```python
from build123d import *

# Parameters (mm, degrees)
F0_W     = 76.2
F0_H     = 50.8
F1_DEPTH = 2.54
F2_W     = 71.12
F2_H     = 45.72
F3_DEPTH = 2.54
F4_W     = 33.02
F4_H     = 5.08
F5_DEPTH = 2.54
F7_DEPTH = 2.54
F9_DEPTH = 25.4


with BuildPart() as f1:
    # F0 (on Top) → F1 (new body)
    with BuildSketch(Plane.XY):
        with Locations((13.626695, -1.068337)):
            Rectangle(F0_W, F0_H)
    extrude(amount=F1_DEPTH)

    # F2 (on face) → F3 (join)
    with BuildSketch(Plane.XY.offset(2.54)):
        with Locations((13.626695, -1.068337)):
            Rectangle(F2_W, F2_H)
    extrude(amount=F3_DEPTH)

    # F4 (on face) → F5 (join)
    with BuildSketch(Plane.XY.offset(5.08)):
        with Locations((25.056695, -21.388337)):
            Rectangle(F4_W, F4_H)
    extrude(amount=F5_DEPTH)

    # F6 (on face) → F7 (cut)
    with BuildSketch(Plane.XY.offset(5.08)):
        Polygon((44.106695, 16.711663), (-16.853305, 16.711663), (-16.853305, -18.848337), (8.546695, -18.848337), (41.566695, -18.848337), (44.106695, -18.848337), align=None)
    extrude(amount=-F7_DEPTH, mode=Mode.SUBTRACT)

    # F8 (on face) → F9 (cut)
    with BuildSketch(Plane(origin=(0, 0, 0), x_dir=(1, 0, 0), z_dir=(0, 0, -1))):
        with BuildLine():
            Line((13.626695, 13.768337), (13.626695, 16.308337))
            ThreePointArc((13.626695, 16.308337), (11.830644, 15.564388), (11.086695, 13.768337))
            Line((11.086695, 13.768337), (13.626695, 13.768337))
        make_face()
        with BuildLine():
            ThreePointArc((11.086695, 13.768337), (13.626695, 11.228337), (16.166695, 13.768337))
            ThreePointArc((16.166695, 13.768337), (15.422746, 15.564388), (13.626695, 16.308337))
            Line((13.626695, 16.308337), (13.626695, 13.768337))
            Line((13.626695, 13.768337), (11.086695, 13.768337))
        make_face()
        with BuildLine():
            Line((13.978975, 1.068088), (13.990214, -1.471887))
            ThreePointArc((13.990214, -1.471887), (15.778995, -0.723985), (16.518975, 1.068088))
            Line((16.518975, 1.068088), (13.978975, 1.068088))
        make_face()
        with BuildLine():
            ThreePointArc((16.518975, 1.068088), (12.178954, 2.860161), (13.990214, -1.471887))
            Line((13.990214, -1.471887), (13.978975, 1.068088))
            Line((13.978975, 1.068088), (16.518975, 1.068088))
        make_face()
        with BuildLine():
            ThreePointArc((14.046408, -14.171265), (14.068887, -14.171564), (14.091368, -14.171663))
            ThreePointArc((14.091368, -14.171663), (15.887419, -13.427715), (16.631368, -11.631663))
            ThreePointArc((16.631368, -11.631663), (15.863418, -9.811927), (14.023935, -9.092559))
            Line((14.023935, -9.092559), (14.046408, -14.171265))
        make_face()
        with BuildLine():
            ThreePointArc((14.023935, -9.092559), (11.551393, -11.642903), (14.046408, -14.171265))
            Line((14.046408, -14.171265), (14.023935, -9.092559))
        make_face()
        with BuildLine():
            Line((26.678975, 1.068088), (26.690214, -1.471887))
            ThreePointArc((26.690214, -1.471887), (28.478995, -0.723985), (29.218975, 1.068088))
            ThreePointArc((29.218975, 1.068088), (26.678975, 3.608088), (24.138975, 1.068088))
            Line((24.138975, 1.068088), (26.678975, 1.068088))
        make_face()
        with BuildLine():
            ThreePointArc((24.138975, 1.068088), (24.886902, -0.731933), (26.690214, -1.471887))
            Line((26.690214, -1.471887), (26.678975, 1.068088))
            Line((26.678975, 1.068088), (24.138975, 1.068088))
        make_face()
    extrude(amount=-F9_DEPTH, mode=Mode.SUBTRACT)


solid = f1.part
```
Geometry: final body of the model. Coordinates: model frame, mm. A direction names the side the tool comes from. Round coordinates to 2 decimals unless told otherwise and drop trailing zeros. Write each loop counter-clockwise with the first axis right and the second up, starting at its lowest first coordinate (ties: lowest second). Pieces come first, ordered by that corner, then holes.
Item 1: Section query A-A (y = 0). Return loops of the section in (x, z).
Item 2: Section query D-D (y = 19.5). Return loops of the section in (x, z), plus the area to 3 significant figures.
Item 3: Pin query (flat end, axial travel): P1, Ø13.5, axis at x = 17.5, y = 7, coming from the +Z side; P2, Ø1.3, axis at y = 8.5, z = 4, coming from the -X side; P3, Ø0.8, axis at y = -6, z = 4.5, coming from the +X side; P4, Ø3, axis at x = 13.98, y = -1.07, coming from the -Z side. Return the tip coordinate at first contact, or that it passes through.
Item 4: Material intervals for L1, parallel to X at y = 8, z = 4; L2, parallel to Y at x = 0, z = 4; L3, parallel to X at y = -3, z = 1.5, sorted ascending.
Item 5: Set-up query: faces 4 (the face through (20, -18.848, 5)), 5 (the face through (8.547, -21, 6)), 6 (the face through (13, -23.928, 4)), 7 (the face through (41.567, -21, 6)). Return all of +Z, -Z, +X, -X, +Y, -Y with unobstructed straight access to the full face (end or side cutting, diameter ignored); none if empty.
Item 6: Section query B-B (x = 15). Return loops of the section in (y, z), plus the area to 3 significant figures.
Item 7: Mould query, pull axis Y, two halves, no side actions, for faces 1 (the face through (44.107, -1, 4)), 2 (the face through (49.187, -1, 4)), 3 (the face through (13, 21.792, 4)). Classes: +Y half, -Y half, draft (parallel to the pull), parting line (faces both ways), or undercut.
Item 8: Section query C-C (z = 0.75). Return loops of the section in (x, y), plus the area to 3 significant figures.
Completed:
1. outline: (-24.47, 0) - (11.67, 0) - (11.67, 2.54) - (-16.85, 2.54) - (-16.85, 5.08) - (-21.93, 5.08) - (-21.93, 2.54) - (-24.47, 2.54) - close; (16.28, 0) - (24.37, 0) - (24.37, 2.54) - (16.28, 2.54) - close; (28.98, 0) - (51.73, 0) - (51.73, 2.54) - (49.19, 2.54) - (49.19, 5.08) - (44.11, 5.08) - (44.11, 2.54) - (28.98, 2.54) - close
2. outline: (-24.47, 0) - (51.73, 0) - (51.73, 2.54) - (49.19, 2.54) - (49.19, 5.08) - (-21.93, 5.08) - (-21.93, 2.54) - (-24.47, 2.54) - close
2. area: 374 mm2
3. P1: stops at z = 2.54
3. P2: stops at x = -21.93
3. P3: stops at x = 49.19
3. P4: passes through
4. L1: x = -21.93 to -16.85, 44.11 to 49.19
4. L2: y = -23.93 to -18.85, 16.71 to 21.79
4. L3: x = -24.47 to 12.33, 15.63 to 25.03, 28.33 to 51.73
5. face 4: +Z
5. face 5: +Z, -X, +Y, -Y
5. face 6: +Z, +X, -X, -Y
5. face 7: +Z, +X, +Y, -Y
6. outline: (-26.47, 0) - (-15.91, 0) - (-15.91, 2.54) - (-18.85, 2.54) - (-18.85, 7.62) - (-23.93, 7.62) - (-23.93, 2.54) - (-26.47, 2.54) - close; (-11.63, 0) - (-3.39, 0) - (-3.39, 2.54) - (-11.63, 2.54) - close; (1.26, 0) - (9.26, 0) - (9.26, 2.54) - (1.26, 2.54) - close; (14, 0) - (24.33, 0) - (24.33, 2.54) - (21.79, 2.54) - (21.79, 5.08) - (16.71, 5.08) - (16.71, 2.54) - (14, 2.54) - close
6. area: 133 mm2
7. face 1: undercut
7. face 2: draft
7. face 3: +Y half
8. outline: (-24.47, -26.47) - (51.73, -26.47) - (51.73, 24.33) - (-24.47, 24.33) - close; hole circle Ø5.08 at (13.98, -1.07); hole (13.63, -16.31) arc R2.54 ccw to (16.17, -13.77) arc R2.54 ccw (long way) to start; hole (14.02, 9.09) arc R2.54 ccw to (16.63, 11.63) arc R2.54 ccw to (14.09, 14.17) arc R2.53 ccw to (14.05, 14.17) arc R2.54 ccw to start; hole (26.69, 1.47) arc R2.54 ccw (long way) to (29.22, -1.07) arc R2.54 ccw to start
8. area: 3,790 mm2
